Check sheet for the modelled part. Datum: model origin and axes. Units: mm. Give positions to 0.01 mm unless a question says otherwise; leave off trailing zeros. Order: outer loops, then holes, each group sorted by start corner. A loop starts at its lowest first (then second) coordinate and runs counter-clockwise, first axis right, second up.
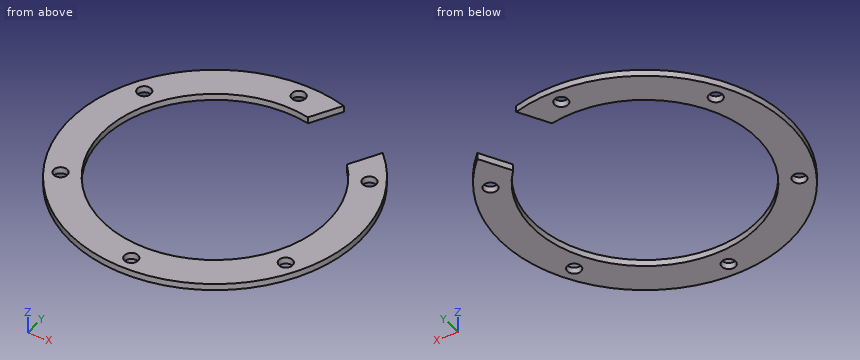
from build123d import *

# Parameters (mm, degrees)
SKETCH_1_R          = 44.5
SKETCH_1_R_2        = 34.5
EXTRUDE_1_DEPTH     = 2
SKETCH_2_R          = 2.1
CUT_EXTRUDE_1_DEPTH = 26
CUT_EXTRUDE_2_DEPTH = 26


with BuildPart() as part:
    # 草图1 → 凸台-拉伸1 (new body)
    with BuildSketch(Plane.XY):
        Circle(SKETCH_1_R)
        Circle(SKETCH_1_R_2, mode=Mode.SUBTRACT)
    extrude(amount=EXTRUDE_1_DEPTH)

    # 草图2 → 切除-拉伸1 (cut)
    with BuildSketch(Plane.XY.offset(2)):
        with Locations((0, 40)):
            Circle(SKETCH_2_R)
        with Locations((34.641016151, 20)):
            Circle(SKETCH_2_R)
        with Locations((34.641016151, -20)):
            Circle(SKETCH_2_R)
        with Locations((0, -40)):
            Circle(SKETCH_2_R)
        with Locations((-34.641016151, -20)):
            Circle(SKETCH_2_R)
        with Locations((-34.641016151, 20)):
            Circle(SKETCH_2_R)
    extrude(amount=-CUT_EXTRUDE_1_DEPTH, mode=Mode.SUBTRACT)

    # 草图3 → 切除-拉伸2 (cut)
    with BuildSketch(Plane.XY.offset(2)):
        Polygon((-6.056039584, 11.510631748), (15.427420122, 48.721075481), (34.479979005, 37.721075481), (12.996519299, 0.510631748), align=None)
    extrude(amount=-CUT_EXTRUDE_2_DEPTH, mode=Mode.SUBTRACT)


solid = part.part
1) Section check D-D, the plane y = 20. Record the cut outline in (x, z), then the cut area to 3 significant figures.
Recorded:
outline: (-39.75, 0) - (-36.74, 0) - (-36.74, 2) - (-39.75, 2) - close; (-32.54, 0) - (-28.11, 0) - (-28.11, 2) - (-32.54, 2) - close; (28.11, 0) - (32.54, 0) - (32.54, 2) - (28.11, 2) - close; (36.74, 0) - (39.75, 0) - (39.75, 2) - (36.74, 2) - close
area: 29.8 mm2
2) Section check C-C, the plane z = 1.6. Record the cut outline in (x, y).
Recorded:
outline: (6.82, 33.82) - (12.03, 42.84) arc R44.5 ccw (long way) to (31.09, 31.84) - (25.88, 22.82) arc R34.5 cw (long way) to start; hole circle Ø4.2 at (-34.64, -20); hole circle Ø4.2 at (-34.64, 20); hole circle Ø4.2 at (0, -40); hole circle Ø4.2 at (0, 40); hole circle Ø4.2 at (34.64, -20); hole circle Ø4.2 at (34.64, 20)
3) Depth check by flat-ended pin: pin 1 Ø3 at (x, y) = (-35, -26.5) entering from -Z; pin 2 Ø1 at (y, z) = (2, 0.5) entering from -X. Enter the tip coordinate at first touch or a pass-through.
Recorded:
pin 1: stops at z = 0
pin 2: stops at x = -44.47
4) Section check B-B, the plane x = 29. Record the cut outline in (y, z).
Recorded:
outline: (-33.75, 0) - (-18.69, 0) - (-18.69, 2) - (-33.75, 2) - close; (18.69, 0) - (28.23, 0) - (28.23, 2) - (18.69, 2) - close
5) Section check A-A, the plane y = -40. Record the cut outline in (x, z).
Recorded:
outline: (-19.5, 0) - (-2.1, 0) - (-2.1, 2) - (-19.5, 2) - close; (2.1, 0) - (19.5, 0) - (19.5, 2) - (2.1, 2) - close
6) Material ranges on L1, parallel to Y at x = 0, z = 1.6; L2, parallel to X at y = -1, z = 1.3; L3, parallel to Y at x = -8.5, z = 0.2, recorded low to high.
Recorded:
L1: y = -44.5 to -42.1, -37.9 to -34.5, 34.5 to 37.9, 42.1 to 44.5
L2: x = -44.49 to -34.49, 34.49 to 44.49
L3: y = -43.68 to -33.44, 33.44 to 43.68
